Geometry: final body of the model. Coordinates: model frame, mm. Round coordinates to 2 decimals unless told otherwise and drop trailing zeros. Order: outer loops, then holes, each group sorted by start corner. A loop starts at its lowest first (then second) coordinate and runs counter-clockwise, first axis right, second up. Notation, with made-up numbers: (3, 13) - (17, 13) arc R12 ccw to (17, 18) - close; hole circle Ø3 at (59, 63.25). An arc over 180 degrees is marked (long way). Put each result on its own line as item: value. Start each with the question number.
(1) Material intervals for L1, parallel to Y at x = 0, z = 0.9; L2, parallel to X at y = -1, z = 0.6; L3, parallel to X at y = -1.25, z = 1.05, sorted ascending. Write a range as [from, to].
(2) Pull-direction query (X, two-part tool) for faces 1 (the face through (25, 0, 2)), 2 (the face through (1.617, -0.67, 0.986)), 3 (the face through (-5, 0, 1)); classes: released by +X, released by -X, zero draft, split by the parting line, or undercut.
(3) Section A-A (y = -2.5). Output: boundary loops of the cut face in (x, z).
(4) Pin query (flat end, axial travel): P1, Ø3, axis at x = 50, y = 0.02, coming from the +Z side; P2, Ø1, axis at y = 3.5, z = 1, coming from the -X side. Return the tip coordinate at first contact, or that it passes through.
from build123d import *

# Parameters (mm, degrees)
F0_R     = 1.75
F1_DEPTH = 2


with BuildPart() as f1:
    # F0 (on Top) → F1 (new body)
    with BuildSketch(Plane.XY):
        with BuildLine():
            add(Edge.make_bspline(
                [(0, 5), (0.3879096976, 4.9541997763), (0.7758195621, 4.9083974868), (1.1637210766, 4.8626899198)],
                knots=[0, 0, 0, 0, 0.0229747267, 0.0229747267, 0.0229747267, 0.0229747267], degree=3))
            ThreePointArc((0, 5), (-5, 0), (0, -5))
            add(Edge.make_bspline(
                [(0, -5), (0.3884219151, -4.9540765878), (0.7768439434, -4.9081517555), (1.1652569528, -4.8623221031)],
                knots=[0, 0, 0, 0, 0.0230119064, 0.0230119064, 0.0230119064, 0.0230119064], degree=3))
            ThreePointArc((1.1652569528, -4.8623221031), (3.9259575115, -3.0962651078), (5, 0))
            ThreePointArc((5, 0), (3.9254684678, 3.0968850977), (1.1637210766, 4.8626899198))
        make_face()
        Circle(F0_R, mode=Mode.SUBTRACT)
        with BuildLine():
            add(Edge.make_bspline(
                [(1.1637210766, 4.8626899198), (9.2762111087, 3.9067715533), (25.2735349116, 2.1026460012), (40.9534234423, 3.9056306073), (48.6808792271, 4.8436985253)],
                knots=[0.0229747267, 0.0229747267, 0.0229747267, 0.0229747267, 0.5034632902, 0.9708949207, 0.9708949207, 0.9708949207, 0.9708949207], degree=3))
            ThreePointArc((1.1637210766, 4.8626899198), (3.9254684678, 3.0968850977), (5, 0))
            ThreePointArc((5, 0), (3.9259575115, -3.0962651078), (1.1652569528, -4.8623221031))
            add(Edge.make_bspline(
                [(1.1652569528, -4.8623221031), (9.2793010918, -3.9049292925), (25.3078629948, -2.0948602578), (40.9958544704, -3.8869187833), (48.7415823678, -4.8182057098)],
                knots=[0.0230119064, 0.0230119064, 0.0230119064, 0.0230119064, 0.5037363411, 0.9731005035, 0.9731005035, 0.9731005035, 0.9731005035], degree=3))
            ThreePointArc((48.7415823678, -4.8182057098), (45.0000943344, -0.0105696626), (48.6808792271, 4.8436985253))
        make_face()
        with BuildLine():
            add(Edge.make_bspline(
                [(48.6808792271, 4.8436985253), (49.1620366811, 4.9021082249), (49.6431766931, 4.9607078729), (50.1243168109, 5.0192975561)],
                knots=[0.9708949207, 0.9708949207, 0.9708949207, 0.9708949207, 1, 1, 1, 1], degree=3))
            ThreePointArc((48.6808792271, 4.8436985253), (45.0000943344, -0.0105696626), (48.7415823678, -4.8182057098))
            add(Edge.make_bspline(
                [(48.7415823678, -4.8182057098), (49.1854939332, -4.8715782324), (49.629390795, -4.9251017483), (50.0732877564, -4.9786194279)],
                knots=[0.9731005035, 0.9731005035, 0.9731005035, 0.9731005035, 1, 1, 1, 1], degree=3))
            ThreePointArc((50.0732877564, -4.9786194279), (53.5613479622, -3.488682203), (54.9999956555, 0.02084337))
            ThreePointArc((54.9999956555, 0.02084337), (53.5792138507, 3.5121464379), (50.1243168109, 5.0192975561))
        make_face()
        with Locations((49.9999956555, 0.02084337)):
            Circle(F0_R, mode=Mode.SUBTRACT)
    extrude(amount=F1_DEPTH)


solid = f1.part
Checks:
1. L1: y = [-5, -1.75], [1.75, 5]
1. L2: x = [-4.9, -1.44], [1.44, 48.58], [51.42, 54.89]
1. L3: x = [-4.84, -1.22], [1.22, 48.8], [51.2, 54.84]
2. face 1: zero draft
2. face 2: undercut
2. face 3: released by -X
3. outline: (-4.33, 0) - (54.32, 0) - (54.32, 2) - (-4.33, 2) - close
4. P1: passes through
4. P2: stops at x = -4
